```python
from build123d import *

# Parameters (mm, degrees)
SKETCH1_R           = 80
SKETCH1_R_2         = 32.5
BOSS_EXTRUDE1_DEPTH = 4
SKETCH2_R           = 2.6
CUT_EXTRUDE1_DEPTH  = 114.207773585
SKETCH3_R           = 34.5
SKETCH3_R_2         = 32.5
BOSS_EXTRUDE2_DEPTH = 3
CHAMFER1_SIZE       = 3


with BuildPart() as part:
    # Sketch1 → Boss-Extrude1 (new body)
    with BuildSketch(Plane(origin=(0, 0, 0), x_dir=(1, 0, 0), z_dir=(0, 1, 0))):
        with Locations(Location((0, 0, 0), (0, 0, 270))):
            Circle(SKETCH1_R)
        with Locations(Location((0, 0, 0), (0, 0, 270))):
            Circle(SKETCH1_R_2, mode=Mode.SUBTRACT)
    extrude(amount=BOSS_EXTRUDE1_DEPTH)

    # Sketch2 → Cut-Extrude1 (cut, through all)
    with BuildSketch(Plane(origin=(0, 4, 0), x_dir=(1, 0, 0), z_dir=(0, 1, 0))):
        with Locations(Location((0, 73, 0), (0, 0, 270))):
            Circle(SKETCH2_R)
        with Locations(Location((73, 0, 0), (0, 0, 270))):
            Circle(SKETCH2_R)
        with Locations(Location((0, -73, 0), (0, 0, 270))):
            Circle(SKETCH2_R)
        with Locations(Location((-73, 0, 0), (0, 0, 270))):
            Circle(SKETCH2_R)
    extrude(amount=-CUT_EXTRUDE1_DEPTH, mode=Mode.SUBTRACT)

    # Sketch3 → Boss-Extrude2 (add)
    with BuildSketch(Plane(origin=(0, 4, 0), x_dir=(1, 0, 0), z_dir=(0, 1, 0))):
        with Locations(Location((0, 0, 0), (0, 0, 270))):
            Circle(SKETCH3_R)
        with Locations(Location((0, 0, 0), (0, 0, 270))):
            Circle(SKETCH3_R_2, mode=Mode.SUBTRACT)
    extrude(amount=BOSS_EXTRUDE2_DEPTH)

    # Chamfer1
    chamfer1_edges = [part.edges().sort_by_distance(p)[0] for p in [
        (0, 4, -34.5),
    ]]
    chamfer(chamfer1_edges, length=CHAMFER1_SIZE - 0.0001)  # a hair under: the kernel refuses the full size


solid = part.part
```
Geometry check sheet. Reference: the model listing, model coordinates, mm. Coordinates: 2 decimals unless noted, no trailing zeros. Loops run counter-clockwise (first coordinate to the right, second up) from the corner with the lowest first, then second, coordinate; pieces in that order, holes last. Notation, with made-up numbers: (-28.5, 80) -> (-21.5, 80) arc R32 ccw to (-21.5, 112) -> close; hole circle Ø6 at (83, -6.75). An arc over 180 degrees is marked (long way). Put each result on its own line as item: value.
1) Cross-section at D-D on z = -73. Record the boundary of the cut face in (x, y).
Result set:
outline: (-32.73, 0) -> (-2.6, 0) -> (-2.6, 4) -> (-32.73, 4) -> close; (2.6, 0) -> (32.73, 0) -> (32.73, 4) -> (2.6, 4) -> close
2) Release check for a two-part mould opening along X. For faces 1 (the cylindrical face through (0.1, 2, 70.4)), 2 (the cylindrical face through (9.76, 3.45, 31)), 3 (the cylindrical face through (-78.1, 1.97, -17.34)), 4 (the flat face through (-17, 4, 34)) record: released by +X, released by -X, zero draft, split by the parting line, or undercut.
Result set:
face 1: undercut
face 2: undercut
face 3: split by the parting line
face 4: zero draft
3) Thickness scan on line 1 (X direction, y = 2.8, z = 0); line 2 (Y direction, x = 54.5, z = -57.5); line 3 (Z direction, x = -14, y = 6.5). Record the ranges inside material, lowest first.
Result set:
line 1: x = -80 to -75.6, -70.4 to -32.5, 32.5 to 70.4, 75.6 to 80
line 2: y = 0 to 4
line 3: z = -32.08 to -29.33, 29.33 to 32.08
4) Cross-section at C-C on y = 1.75. Record the boundary of the cut face in (x, z), plus the area to 3 significant figures.
Result set:
outline: circle Ø160 at (0, 0); hole circle Ø5.2 at (-73, 0); hole circle Ø65 at (0, 0); hole circle Ø5.2 at (0, -73); hole circle Ø5.2 at (0, 73); hole circle Ø5.2 at (73, 0)
area: 16,700 mm^2
5) Gauge pin test, flat ends, axial feed: pin 1 Ø1 at (y, z) = (3.5, 28) entering from -X; pin 2 Ø10 at (x, z) = (-26, 34.5) entering from +Y; pin 3 Ø3 at (x, y) = (54, 3) entering from -Z. Record the tip position at first contact, or that the pin passes through.
Result set:
pin 1: stops at x = -75.12
pin 2: stops at y = 4
pin 3: stops at z = -60.36
6) Cross-section at A-A on x = 0. Count the separate pieces of the cut face and the enclosed holes in it, plus the area to 3 significant figures.
Result set:
separate pieces: 4
enclosed holes: 0
area: 359 mm^2
